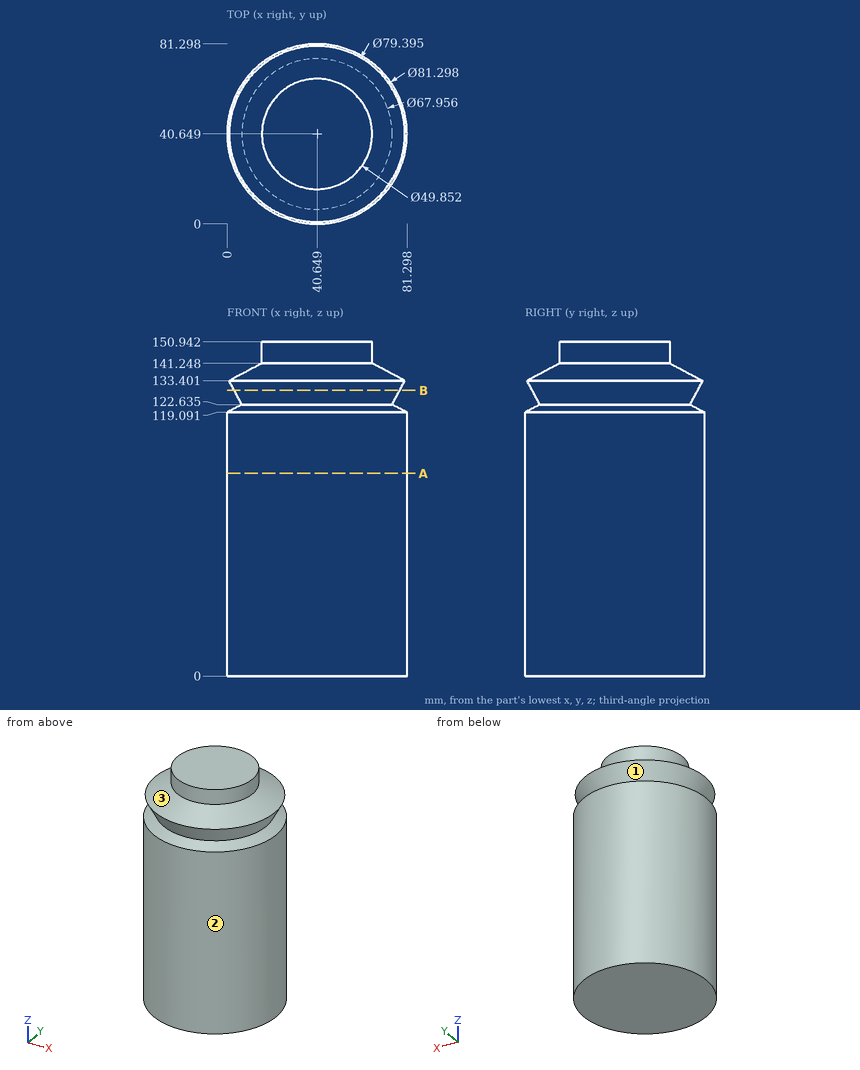
The drawing under review shows one solid part. Ordinate dimensions are in mm from its lowest x, y, z. Give positions to 0.01 mm unless a question says otherwise; leave off trailing zeros. Order: outer loops, then holes, each group sorted by start corner. A loop starts at its lowest first (then second) coordinate and runs counter-clockwise, first axis right, second up. Notation, with made-up numbers: (38.25, 57.5) - (63.25, 57.5) arc R26 cw to (63.25, 71.5) - close; hole circle Ø10 at (-20.5, -35.5). An arc over 180 degrees is marked (long way). Answer as a JSON object with one key per item and string values. Group by question number.
Item 1: Wall thickness on line 1 along Y through (x, z) = (39, 110) (1 decimal); line 2 along Z through (x, y) = (65.5, 13) (1 decimal); line 3 along Z through (x, y) = (77.5, 33) (1 decimal): over which ranges is each line inside the solid? List them lowest first.
Item 2: Clearance check with flat-ended pins moving along their axes: pin 1 Ø1.5 at (x, y) = (66.5, 65) entering from +Z; pin 2 Ø4 at (x, y) = (46.5, 72.5) entering from +Z; pin 3 Ø4 at (y, z) = (30.5, 44) entering from -X (1 decimal). State where each tip first meets the part, or that it passes through.
Item 3: Take a section at A-A on z = 91.5. Give the boundary of the cut face in (x, y).
Item 4: Draft analysis for pull direction Z (two halves, no side actions). For the marked faces 1, 2 and 3, state which applies: pulls with the +Z half, pulls with the -Z half, needs draft (parallel to the pull), parting line crosses it, or undercut.
Item 5: Take a section at B-B on z = 129. Give the boundary of the cut face in (x, y).
Reported:
{
 "1": {"line 1": "0 to 81.3", "line 2": "0 to 120.9, 128.7 to 134.7", "line 3": "0 to 120.7, 129.5 to 134.5"},
 "2": {"pin 1": "z = 136.02", "pin 2": "z = 138.35", "pin 3": "x = 0.8"},
 "3": {"outline": "circle Ø81.3 at (40.65, 40.65)"},
 "4": {"face 1": "undercut", "face 2": "needs draft", "face 3": "pulls with the +Z half"},
 "5": {"outline": "circle Ø74.72 at (40.65, 40.65)"}
}
